Here's the drawing with two shaded views (mm, measured from the low corner). I have some questions. Coordinates: 2 decimals unless noted, no trailing zeros. Write each loop counter-clockwise with the first axis right and the second up, starting at its lowest first coordinate (ties: lowest second). Pieces come first, ordered by that corner, then holes. Notation, with made-up numbers: (35, 51.5) -> (55, 51.5) arc R22 ccw to (55, 69.5) -> close; hole circle Ø10 at (-19.5, 63). An arc over 180 degrees is marked (long way). Put each result on its own line as item: value.
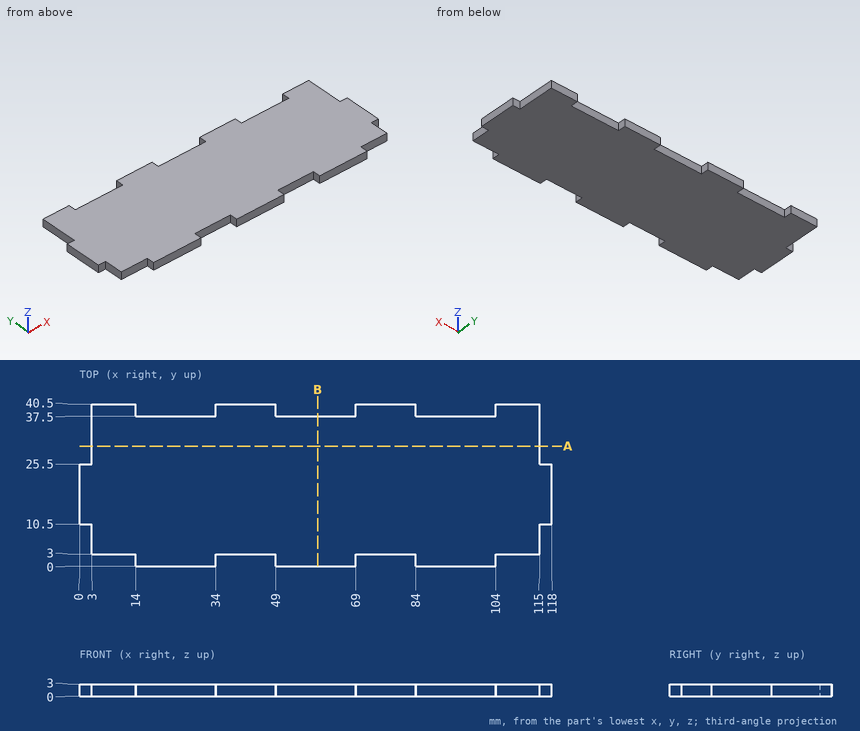
Item 1: Imagine slicing it at B-B on x = 59.5. Write out the boundary of the cut face in (y, z), then the cut area to 4 significant figures.
Output:
outline: (0, 0) -> (37.5, 0) -> (37.5, 3) -> (0, 3) -> close
area: 112.5 mm²
Item 2: Imagine slicing it at A-A on y = 30. Write out the boundary of the cut face in (x, z), then the cut area to 3 significant figures.
Output:
outline: (3, 0) -> (115, 0) -> (115, 3) -> (3, 3) -> close
area: 336 mm²
Item 3: For P1, Ø0.9, axis at x = 116.5, z = 1, coming from the -Y side; P2, Ø0.9, axis at y = 1.5, z = 2, coming from the +X side; P3, Ø1.5, axis at y = 28, z = 2, coming from the +X side, each with a flat end and sliding along its axis, tell me the tip position at first contact or that it passes through.
Output:
P1: stops at y = 10.5
P2: stops at x = 104
P3: stops at x = 115
Item 4: Please list where these lines run through material, in increasing order: line 1 along X through (y, z) = (38, 2.85); line 2 along Y through (x, z) = (82, 0.9); line 3 along Y through (x, z) = (66.5, 1.4). Write a range as from..to.
Output:
line 1: x = 3..14, 34..49, 69..84, 104..115
line 2: y = 3..40.5
line 3: y = 0..37.5
